from build123d import *

# Parameters (mm, degrees)
SKETCH1_W           = 45.25
SKETCH1_H           = 44
SKETCH1_W_2         = 37.25
SKETCH1_H_2         = 36
EXTRUDE_THIN1_DEPTH = 250
SKETCH2_R           = 4
CUT_EXTRUDE1_DEPTH  = 45


with BuildPart() as part:
    # Sketch1 → Extrude-Thin1 (new body, symmetric)
    with BuildSketch(Plane.XY):
        Rectangle(SKETCH1_W, SKETCH1_H)
        Rectangle(SKETCH1_W_2, SKETCH1_H_2, mode=Mode.SUBTRACT)
    extrude(amount=EXTRUDE_THIN1_DEPTH, both=True)

    # Sketch2 → Cut-Extrude1 (cut, through all)
    with BuildSketch(Plane(origin=(0, 22, 0), x_dir=(1, 0, 0), z_dir=(0, 1, 0))):
        with Locations((0, 217.131701203)):
            Circle(SKETCH2_R)
        with Locations((0, -222.868298797)):
            Circle(SKETCH2_R)
    extrude(amount=-CUT_EXTRUDE1_DEPTH, mode=Mode.SUBTRACT)


solid = part.part
Work out the finished part from the listing and answer in its coordinate system (mm). A direction names the side the tool comes from. Coordinates: 2 decimals unless noted, no trailing zeros. Write each loop counter-clockwise with the first axis right and the second up, starting at its lowest first coordinate (ties: lowest second). Pieces come first, ordered by that corner, then holes. Notation, with made-up numbers: (37.5, -38.75) - (94.5, -38.75) arc R23 ccw to (94.5, -19.75) - close; hole circle Ø4 at (80.25, -25.5). An arc over 180 degrees is marked (long way). One line per question, with ' | ' between items.
1) Find section C-C, the plane z = 146.5. Determine the outline of the cut face in (x, y) (3 decimals), and give its area (3 significant figures).
Checks:
outline: (-22.625, -22) - (22.625, -22) - (22.625, 22) - (-22.625, 22) - close; hole (-18.625, -18) - (18.625, -18) - (18.625, 18) - (-18.625, 18) - close | area: 650 mm2
2) For faces 4 (the face through (18.625, 0, 4)), 5 (the face through (-0.5, 20, 218.9)), determine the directions among +Z, -Z, +X, -X, +Y, -Y from which every point of the face is accessible in a straight line to the end or side of a thin tool.
Checks:
face 4: +Z, -Z | face 5: +Y, -Y
3) The mould has two halves that part along Y. Classify faces 1 (the face through (0, 22, 4)), 2 (the face through (-0.5, -20, -221.1)), 3 (the face through (0, 18, 4)): +Y half, -Y half, draft (parallel to the pull), parting line (faces both ways), or undercut.
Checks:
face 1: +Y half | face 2: draft | face 3: undercut
4) Find section A-A, the plane x = -9.5. Determine the outline of the cut face in (y, z), and give its area (3 significant figures).
Checks:
outline: (-22, -250) - (-18, -250) - (-18, 250) - (-22, 250) - close; (18, -250) - (22, -250) - (22, 250) - (18, 250) - close | area: 4,000 mm2
5) Consider probe 1 along Z at (x, y) = (0, -21); probe 2 along X at (y, z) = (-3.5, 217.5) (3 decimals); probe 3 along Y at (x, z) = (7, -63.5). Determine where each line is inside the solid, lowest interval first. Write a range as [from, to].
Checks:
probe 1: [-250, -221.13], [-213.13, 218.87], [226.87, 250] | probe 2: [-22.625, -18.625], [18.625, 22.625] | probe 3: [-22, -18], [18, 22]
6) Find section B-B, the plane y = 1.5. Determine the outline of the cut face in (x, z) (3 decimals).
Checks:
outline: (-22.625, -250) - (-18.625, -250) - (-18.625, 250) - (-22.625, 250) - close; (18.625, -250) - (22.625, -250) - (22.625, 250) - (18.625, 250) - close
